```python
from build123d import *

# Parameters (mm, degrees)
F0_W          = 101.6
F0_H          = 50.8
F1_DEPTH      = 3.175
F5_DEPTH      = 12.7
F5_DEPTH_BACK = 12.7
F8_W          = 101.6
F8_H          = 101.6
F9_DEPTH      = 3.175


with BuildPart() as f1:
    # F0 (on Top) → F1 (new body)
    with BuildSketch(Plane.XY):
        with Locations((50.8, 25.4)):
            Rectangle(F0_W, F0_H)
    extrude(amount=F1_DEPTH)

    # F4 (on plane+point) → F5 (join, two sides)
    with BuildSketch(Plane.YZ.offset(50.8)) as f5_sk:
        with BuildLine():
            ThreePointArc((60.96, 13.335), (57.9842048969, 6.1507951031), (50.8, 3.175))
            Line((50.8, 3.175), (50.8, 0))
            ThreePointArc((50.8, 0), (60.2292689271, 3.9057310729), (64.135, 13.335))
            Line((64.135, 13.335), (60.96, 13.335))
        make_face()
    extrude(amount=F5_DEPTH)
    extrude(f5_sk.sketch, amount=-F5_DEPTH_BACK)

    # F8 (on plane+point) → F9 (join)
    with BuildSketch(Plane.XZ.offset(-60.96)):
        with Locations((50.8, 64.135)):
            Rectangle(F8_W, F8_H)
    extrude(amount=-F9_DEPTH)


solid = f1.part
```
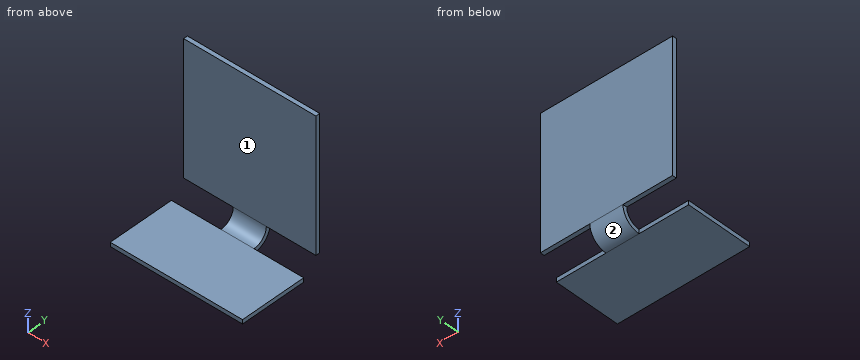
Can you work these out from the model? Positions are in its coordinate system, mm. Face numbers are marked on the shaded views. A direction names the side the tool comes from. Give positions to 0.01 mm unless a question says otherwise; leave off trailing zeros. Write each loop counter-clockwise with the first axis right and the second up, starting at its lowest first coordinate (ties: lowest second). Pieces come first, ordered by that corner, then holes. Notation, with made-up numbers: (49, 23.25) - (60, 23.25) arc R7 ccw to (60, 28.25) - close; hole circle Ø9 at (-21.5, -5). An arc over 180 degrees is marked (long way). Write item = value, one per line. Start each with the question number.
1. Imagine slicing it at B-B (x = 44.5). Please give me the cut outline in (y, z) (3 decimals).
2. Imagine slicing it at C-C (y = 31). Please give me the cut outline in (x, z) (3 decimals), and give its area (3 significant figures).
3. Please list where these lines run through material, in increasing order: line 1 (Y direction, x = 88, z = 108.5) (3 decimals); line 2 (Z direction, x = 41, y = 37.5) (3 decimals).
4. On a 3-axis mill with a long thin cutter (end or side, diameter ignored), from which of +Z, -Z, +X, -X, +Y, -Y can I reach the whole of each face in a straight line? I mean the marked faces 1 and 2. Say none if no direction works.
5. Imagine slicing it at D-D (z = 25.5). Please give me the cut outline in (x, y) (3 decimals), and give its area (3 significant figures).
6. For pin 1 (3.5 mm diameter, centred on x = 85.5, y = 63.5, fed in from -Z) (3 decimals); pin 2 (2 mm diameter, centred on x = 52.5, y = 45, fed in from +Z) (3 decimals); pin 3 (3.5 mm diameter, centred on x = 12, z = 2, fed in from +Y), each with a flat end and sliding along its axis, tell me the tip position at first contact or that it passes through.
7. Imagine slicing it at A-A (x = 9). Please give me the cut outline in (y, z) (3 decimals).
Worked answers:
q1.outline = (0, 0) - (50.8, 0) arc R13.335 ccw to (64.135, 13.335) - (64.135, 114.935) - (60.96, 114.935) - (60.96, 13.335) arc R10.16 cw to (50.8, 3.175) - (0, 3.175) - close
q2.outline = (0, 0) - (101.6, 0) - (101.6, 3.175) - (0, 3.175) - close
q2.area = 323 mm2
q3.line_1 = 60.96 to 64.135
q3.line_2 = 0 to 3.175
q4.face_1 = +Z, +X, -X, -Y
q4.face_2 = -Z, +X, -X, +Y
q5.outline = (0, 60.96) - (101.6, 60.96) - (101.6, 64.135) - (0, 64.135) - close
q5.area = 323 mm2
q6.pin_1 = 13.335
q6.pin_2 = 3.175
q6.pin_3 = 50.8
q7.outline = (0, 0) - (50.8, 0) - (50.8, 3.175) - (0, 3.175) - close; (60.96, 13.335) - (64.135, 13.335) - (64.135, 114.935) - (60.96, 114.935) - close
